Here's how the part is built. I have some questions about the finished solid (model axes, mm). A direction names the side the tool comes from. Coordinates: 2 decimals unless noted, no trailing zeros. Order: outer loops, then holes, each group sorted by start corner. A loop starts at its lowest first (then second) coordinate and runs counter-clockwise, first axis right, second up.
```python
from build123d import *

# Parameters (mm, degrees)
SKETCH1_R           = 0.9
SKETCH1_R_2         = 1.449813
SKETCH1_W           = 3.400011
SKETCH1_H           = 6.165
BOSS_EXTRUDE1_DEPTH = 5.85


with BuildPart() as part:
    # Sketch1 → Boss-Extrude1 (new body)
    with BuildSketch(Plane.XY):
        with BuildLine():
            Line((588.919699582, 440.365819013), (585.919699582, 440.365819013))
            ThreePointArc((585.919699582, 440.365819013), (580.919699582, 435.365819013), (585.919699582, 430.365819013))
            Line((585.919699582, 430.365819013), (588.919699582, 430.365819013))
            ThreePointArc((588.919699582, 430.365819013), (599.557918625, 427.682003659), (607.649897061, 420.272924481))
            ThreePointArc((607.649897061, 420.272924481), (614.550865316, 418.451224777), (615.634267587, 425.505882259))
            ThreePointArc((615.634267587, 425.505882259), (610.653294544, 429.857960207), (604.521800574, 432.33897948))
            ThreePointArc((604.521800574, 432.33897948), (602.091309675, 435.365819013), (604.521800574, 438.392658547))
            ThreePointArc((604.521800574, 438.392658547), (610.653294544, 440.87367782), (615.634267587, 445.225755768))
            ThreePointArc((615.634267587, 445.225755768), (614.550865316, 452.28041325), (607.649897061, 450.458713546))
            ThreePointArc((607.649897061, 450.458713546), (599.557918625, 443.049634368), (588.919699582, 440.365819013))
        make_face()
        with Locations((611.919699582, 448.265819013)):
            Circle(SKETCH1_R, mode=Mode.SUBTRACT)
        with Locations((611.919699582, 422.465819013)):
            Circle(SKETCH1_R, mode=Mode.SUBTRACT)
        with Locations((588.919699582, 435.365819013)):
            Circle(SKETCH1_R_2, mode=Mode.SUBTRACT)
        with Locations((594.169518082, 435.365819013)):
            Rectangle(SKETCH1_W, SKETCH1_H, mode=Mode.SUBTRACT)
    extrude(amount=BOSS_EXTRUDE1_DEPTH)


solid = part.part
```
Q1. If we section it at C-C on z = 2.35: Write out the boundary of the cut face in (x, y).
Q2. If we section it at A-A on y = 433: Write out the boundary of the cut face in (x, z), then the cut area to 3 significant figures.
Q3. If we section it at B-B on x = 607: Write out the boundary of the cut face in (y, z), then the cut area to 3 significant figures.
Q4. I need wall thicknesses on L1, parallel to Y at x = 612, z = 2.25; L2, parallel to Y at x = 595.5, z = 2; L3, parallel to Y at x = 608, z = 3.05. Which ranges of each line are inside material? Lowest first, please.
Q5. If we section it at D-D on x = 586.5: Write out the boundary of the cut face in (y, z).
Q6. We'd pull the mould along X, two halves only. Please class faces 6 (the cylindrical face through (580.92, 435.48, 2.88)), 7 (the flat face through (592.47, 435, 3)), 8 (the flat face through (587, 430.366, 3)), 9 (the flat face through (594, 432.283, 3)): pulls with the +X half, pulls with the -X half, needs draft (parallel to the pull), parting line crosses it, or undercut.
Q7. For faces 1 (the cylindrical face through (610.574, 440.825, 2.884)), 2 (the flat face through (594, 438.448, 3)), 3 (the flat face through (587, 440.366, 3)), 4 (the cylindrical face through (599.421, 427.755, 2.884)), 5 (the flat face through (599, 436, 0)), which set-ups out of +Z, -Z, +X, -X, +Y, -Y let a thin tool reach every point of the face, with its end or its side?
Q8. Will these pins go through, and if not, where does the flat tip stop? pin 1 (2.5 mm diameter, centred on x = 586.5, z = 4, fed in from -Y); pin 2 (0.9 mm diameter, centred on x = 587, z = 2, fed in from +Y); pin 3 (1 mm diameter, centred on x = 593.5, z = 2, fed in from -Y); pin 4 (1.6 mm diameter, centred on x = 611.92, y = 448.27, fed in from +Z).
Reply:
1. outline: (585.92, 430.37) - (588.92, 430.37) arc R22.43 cw to (607.65, 420.27) arc R4.8 ccw (long way) to (615.63, 425.51) arc R19.92 ccw to (604.52, 432.34) arc R3.1 cw to (604.52, 438.39) arc R19.92 ccw to (615.63, 445.23) arc R4.8 ccw (long way) to (607.65, 450.46) arc R22.43 cw to (588.92, 440.37) - (585.92, 440.37) arc R5 ccw to start; hole circle Ø2.9 at (588.92, 435.37); hole (592.47, 432.28) - (595.87, 432.28) - (595.87, 438.45) - (592.47, 438.45) - close; hole circle Ø1.8 at (611.92, 422.47); hole circle Ø1.8 at (611.92, 448.27)
2. outline: (581.51, 0) - (592.47, 0) - (592.47, 5.85) - (581.51, 5.85) - close; (595.87, 0) - (603.19, 0) - (603.19, 5.85) - (595.87, 5.85) - close
2. area: 107 mm2
3. outline: (421.21, 0) - (431.62, 0) - (431.62, 5.85) - (421.21, 5.85) - close; (439.11, 0) - (449.52, 0) - (449.52, 5.85) - (439.11, 5.85) - close
3. area: 122 mm2
4. L1: y = 417.67 to 421.57, 423.36 to 428.95, 441.78 to 447.37, 449.16 to 453.07
4. L2: y = 429.38 to 432.28, 438.45 to 441.35
4. L3: y = 419.7 to 431.23, 439.5 to 451.04
5. outline: (430.37, 0) - (440.37, 0) - (440.37, 5.85) - (430.37, 5.85) - close
6. face 6: pulls with the -X half
6. face 7: undercut
6. face 8: needs draft
6. face 9: undercut
7. face 1: +Z, -Z, +X
7. face 2: +Z, -Z
7. face 3: +Z, -Z, -X, +Y
7. face 4: +Z, -Z, -X, -Y
7. face 5: -Z, +X, -X, +Y, -Y
8. pin 1: stops at y = 430.37
8. pin 2: stops at y = 440.37
8. pin 3: stops at y = 429.78
8. pin 4: passes through
